The listing builds one solid part. Answer for the finished solid, in the listing's coordinates (mm). A direction names the side the tool comes from. Round coordinates to 2 decimals unless told otherwise and drop trailing zeros. Order: outer loops, then holes, each group sorted by start corner. A loop starts at its lowest first (then second) coordinate and runs counter-clockwise, first axis right, second up. Notation, with made-up numbers: M 66.25,61.5 L 79.25,61.5 A37 cw 79.25,98.5 Z; hole C 45.5,7 d6. An arc over 180 degrees is marked long. Put each result on its own line as item: value. Start each with the question number.
1. The mould has two halves that part along Y. Classify faces 1 (the face through (20, 120, 5)), 2 (the face through (20, 145.1, 3)), 3 (the face through (29.84, 141.34, 2.03)): +Y half, -Y half, draft (parallel to the pull), parting line (faces both ways), or undercut.
2. The part is cut by section A-A (y = 58.5). Give the vertices of the cut face in (x, z), then the cut area to 3 significant figures.
3. Each of these flat-tipped pins is pushed along its axis until it touches: pin 1 Ø1.6 at (y, z) = (55, 0.5) entering from -X; pin 2 Ø2 at (x, y) = (10, 140.1) entering from -Z; pin 3 Ø1.5 at (x, y) = (19, 139.5) entering from +Z. Where does it stop, or does it pass through?
4. The part is cut by section C-C (x = 20). Count the separate pieces of the cut face and the enclosed holes in it, then the cut area to 3 significant figures.
5. Consider line 1 (X direction, y = 140.1, z = 3.1); line 2 (Y direction, x = 20, z = 1.35); line 3 (Y direction, x = 13.5, z = 0.5). Determine where each line is inside the solid, lowest interval first.
6. The part is cut by section B-B (x = 30). Give the vertices of the cut face in (y, z).
7. The part is cut by section D-D (x = 4). Give the vertices of the cut face in (y, z), then the cut area to 3 significant figures.
8. Which of the six approach directions +Z, -Z, +X, -X, +Y, -Y give full straight-line access (tool end or side, diameter ignored) to faces 4 (the face through (18, 121, 7)), 5 (the face through (38, 59, 5)), 6 (the face through (11, 139, 4))?
from build123d import *

# Parameters (mm, degrees)
SKETCH1_W           = 40
SKETCH1_H           = 145.1
BOSS_EXTRUDE1_DEPTH = 7
SKETCH2_R           = 1.25
CUT_EXTRUDE1_DEPTH  = 7
SKETCH3_R           = 2.5
CUT_EXTRUDE2_DEPTH  = 3
SKETCH4_R           = 6.35
CUT_EXTRUDE3_DEPTH  = 8
SKETCH5_W           = 36
SKETCH5_H           = 120
CUT_EXTRUDE4_DEPTH  = 5
SKETCH6_W           = 26
SKETCH6_H           = 12
CUT_EXTRUDE5_DEPTH  = 3


with BuildPart() as part:
    # Sketch1 → Boss-Extrude1 (new body)
    with BuildSketch(Plane.XY):
        with Locations((20, 72.55)):
            Rectangle(SKETCH1_W, SKETCH1_H)
    extrude(amount=BOSS_EXTRUDE1_DEPTH)

    # Sketch2 → Cut-Extrude1 (cut)
    with BuildSketch(Plane.XY.offset(7)):
        with Locations((20, 140.1)):
            Circle(SKETCH2_R)
        with Locations((10, 140.1)):
            Circle(SKETCH2_R)
        with Locations((30, 140.1)):
            Circle(SKETCH2_R)
    extrude(amount=-CUT_EXTRUDE1_DEPTH, mode=Mode.SUBTRACT)

    # Sketch3 → Cut-Extrude2 (cut)
    with BuildSketch(Plane.XY.offset(7)):
        with Locations((10, 140.1)):
            Circle(SKETCH3_R)
        with Locations((20, 140.1)):
            Circle(SKETCH3_R)
        with Locations((30, 140.1)):
            Circle(SKETCH3_R)
    extrude(amount=-CUT_EXTRUDE2_DEPTH, mode=Mode.SUBTRACT)

    # Sketch4 → Cut-Extrude3 (cut, through all)
    with BuildSketch(Plane.XY.offset(7)):
        with Locations((20, 24)):
            Circle(SKETCH4_R)
    extrude(amount=-CUT_EXTRUDE3_DEPTH, mode=Mode.SUBTRACT)

    # Sketch5 → Cut-Extrude4 (cut)
    with BuildSketch(Plane.XY.offset(7)):
        with Locations((20, 60)):
            Rectangle(SKETCH5_W, SKETCH5_H)
    extrude(amount=-CUT_EXTRUDE4_DEPTH, mode=Mode.SUBTRACT)

    # Sketch6 → Cut-Extrude5 (cut, through all)
    with BuildSketch(Plane.XY.offset(2)):
        with Locations((20, 102)):
            Rectangle(SKETCH6_W, SKETCH6_H)
        with Locations((20, 78)):
            Rectangle(SKETCH6_W, SKETCH6_H)
        with Locations((20, 54)):
            Rectangle(SKETCH6_W, SKETCH6_H)
    extrude(amount=-CUT_EXTRUDE5_DEPTH, mode=Mode.SUBTRACT)


solid = part.part
Resolved:
1. face 1: -Y half
1. face 2: +Y half
1. face 3: undercut
2. outline: M 0,0 L 7,0 L 7,2 L 2,2 L 2,7 L 0,7 Z; M 33,0 L 40,0 L 40,7 L 38,7 L 38,2 L 33,2 Z
2. area: 48.0 mm2
3. pin 1: x = 0
3. pin 2: through
3. pin 3: z = 4
4. separate pieces: 6
4. enclosed holes: 0
4. area: 293 mm2
5. line 1: 0 to 8.75, 11.25 to 18.75, 21.25 to 28.75, 31.25 to 40
5. line 2: 0 to 17.65, 30.35 to 48, 60 to 72, 84 to 96, 108 to 138.85, 141.35 to 145.1
5. line 3: 0 to 48, 60 to 72, 84 to 96, 108 to 145.1
6. outline: M 0,0 L 48,0 L 48,2 L 0,2 Z; M 60,0 L 72,0 L 72,2 L 60,2 Z; M 84,0 L 96,0 L 96,2 L 84,2 Z; M 108,0 L 138.85,0 L 138.85,4 L 137.6,4 L 137.6,7 L 120,7 L 120,2 L 108,2 Z; M 141.35,0 L 145.1,0 L 145.1,7 L 142.6,7 L 142.6,4 L 141.35,4 Z
7. outline: M 0,0 L 145.1,0 L 145.1,7 L 120,7 L 120,2 L 0,2 Z
7. area: 416 mm2
8. face 4: +Z, +X, -X, +Y, -Y
8. face 5: +Z, -Y
8. face 6: +Z
